Design review of the part built by this model. Coordinates are the model's own, in mm. Coordinates: 2 decimals unless noted, no trailing zeros. Loops run counter-clockwise (first coordinate to the right, second up) from the corner with the lowest first, then second, coordinate; pieces in that order, holes last. Notation, with made-up numbers: (-15.75, -30.75) -> (9.25, -30.75) arc R27 cw to (9.25, 2.25) -> close; hole circle Ø6 at (8, 16). An arc over 180 degrees is marked (long way). Answer as a JSON object with one key per item and string values.
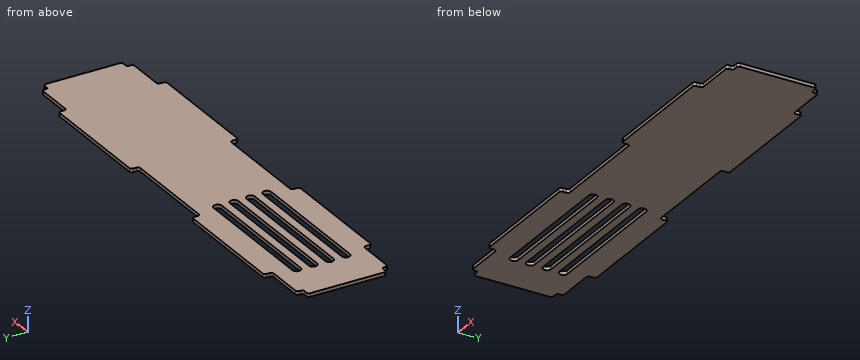
```python
from build123d import *

# Parameters (mm, degrees)
PAD_DEPTH = 1.8542


with BuildPart() as part:
    # Sketch (on Face54 of Binder001) → Pad (new body)
    with BuildSketch(Plane.XY.offset(-14.1418)):
        with BuildLine():
            Line((326.2352, 174.592), (328.0894, 174.592))
            ThreePointArc((329.2894, 173.392), (328.937928, 174.240528), (328.0894, 174.592))
            Line((329.2894, 173.392), (329.2894, 134.7706))
            ThreePointArc((328.0894, 133.5706), (328.937928, 133.922072), (329.2894, 134.7706))
            Line((328.0894, 133.5706), (326.2352, 133.5706))
            ThreePointArc((326.2352, 133.5706), (325.386672, 133.219128), (325.0352, 132.3706))
            Line((325.0352, 131.4813), (325.0352, 132.3706))
            ThreePointArc((323.8352, 130.2813), (324.683728, 130.632772), (325.0352, 131.4813))
            Line((304.7198, 130.2813), (323.8352, 130.2813))
            ThreePointArc((304.7198, 130.2813), (303.871272, 129.929828), (303.5198, 129.0813))
            Line((303.5198, 129.0813), (303.5198, 127.2271))
            ThreePointArc((302.3198, 126.0271), (303.168328, 126.378572), (303.5198, 127.2271))
            Line((241.3778, 126.0271), (302.3198, 126.0271))
            ThreePointArc((240.1778, 127.2271), (240.529272, 126.378572), (241.3778, 126.0271))
            Line((240.1778, 129.0813), (240.1778, 127.2271))
            ThreePointArc((240.1778, 129.0813), (239.826328, 129.929828), (238.9778, 130.2813))
            Line((187.7682, 130.2813), (238.9778, 130.2813))
            ThreePointArc((187.7682, 130.2813), (186.919672, 129.929828), (186.5682, 129.0813))
            Line((186.5682, 129.0813), (186.5682, 127.2271))
            ThreePointArc((185.3682, 126.0271), (186.216728, 126.378572), (186.5682, 127.2271))
            Line((124.6802, 126.0271), (185.3682, 126.0271))
            ThreePointArc((123.4802, 127.2271), (123.831672, 126.378572), (124.6802, 126.0271))
            Line((123.4802, 129.0813), (123.4802, 127.2271))
            ThreePointArc((123.4802, 129.0813), (123.128728, 129.929828), (122.2802, 130.2813))
            Line((122.2802, 130.2813), (103.1648, 130.2813))
            ThreePointArc((101.9648, 131.4813), (102.316272, 130.632772), (103.1648, 130.2813))
            Line((101.9648, 131.4813), (101.9648, 132.3706))
            ThreePointArc((101.9648, 132.3706), (101.613328, 133.219128), (100.7648, 133.5706))
            Line((100.7648, 133.5706), (98.9106, 133.5706))
            ThreePointArc((97.7106, 134.7706), (98.062072, 133.922072), (98.9106, 133.5706))
            Line((97.7106, 134.7706), (97.7106, 173.392))
            ThreePointArc((98.9106, 174.592), (98.062072, 174.240528), (97.7106, 173.392))
            Line((98.9106, 174.592), (100.7648, 174.592))
            ThreePointArc((100.7648, 174.592), (101.613328, 174.943472), (101.9648, 175.792))
            Line((101.9648, 175.792), (101.9648, 176.6813))
            ThreePointArc((103.1648, 177.8813), (102.316272, 177.529828), (101.9648, 176.6813))
            Line((103.1648, 177.8813), (122.2802, 177.8813))
            ThreePointArc((122.2802, 177.8813), (123.128728, 178.232772), (123.4802, 179.0813))
            Line((123.4802, 179.0813), (123.4802, 180.9355))
            ThreePointArc((124.6802, 182.1355), (123.831672, 181.784028), (123.4802, 180.9355))
            Line((124.6802, 182.1355), (185.3682, 182.1355))
            ThreePointArc((186.5682, 180.9355), (186.216728, 181.784028), (185.3682, 182.1355))
            Line((186.5682, 180.9355), (186.5682, 179.0813))
            ThreePointArc((186.5682, 179.0813), (186.919672, 178.232772), (187.7682, 177.8813))
            Line((238.9778, 177.8813), (187.7682, 177.8813))
            ThreePointArc((238.9778, 177.8813), (239.826328, 178.232772), (240.1778, 179.0813))
            Line((240.1778, 179.0813), (240.1778, 180.9355))
            ThreePointArc((241.3778, 182.1355), (240.529272, 181.784028), (240.1778, 180.9355))
            Line((241.3778, 182.1355), (302.3198, 182.1355))
            ThreePointArc((303.5198, 180.9355), (303.168328, 181.784028), (302.3198, 182.1355))
            Line((303.5198, 180.9355), (303.5198, 179.0813))
            ThreePointArc((303.5198, 179.0813), (303.871272, 178.232772), (304.7198, 177.8813))
            Line((304.7198, 177.8813), (323.8352, 177.8813))
            ThreePointArc((325.0352, 176.6813), (324.683728, 177.529828), (323.8352, 177.8813))
            Line((325.0352, 176.6813), (325.0352, 175.792))
            ThreePointArc((325.0352, 175.792), (325.386672, 174.943472), (326.2352, 174.592))
        make_face()
        with BuildLine():
            ThreePointArc((120.6, 143.367014), (118.457143, 141.224157), (120.6, 139.0813))
            Line((120.6, 139.0813), (189.4484, 139.0813))
            ThreePointArc((189.4484, 139.0813), (191.591257, 141.224157), (189.4484, 143.367014))
            Line((120.6, 143.367014), (189.4484, 143.367014))
        make_face(mode=Mode.SUBTRACT)
        with BuildLine():
            ThreePointArc((120.6, 151.938443), (118.457143, 149.795586), (120.6, 147.652729))
            Line((120.6, 147.652729), (189.4484, 147.652729))
            ThreePointArc((189.4484, 147.652729), (191.591257, 149.795586), (189.4484, 151.938443))
            Line((120.6, 151.938443), (189.4484, 151.938443))
        make_face(mode=Mode.SUBTRACT)
        with BuildLine():
            ThreePointArc((120.6, 160.509871), (118.457143, 158.367014), (120.6, 156.224157))
            Line((120.6, 156.224157), (189.4484, 156.224157))
            ThreePointArc((189.4484, 156.224157), (191.591257, 158.367014), (189.4484, 160.509871))
            Line((120.6, 160.509871), (189.4484, 160.509871))
        make_face(mode=Mode.SUBTRACT)
        with BuildLine():
            ThreePointArc((120.6, 169.0813), (118.457143, 166.938443), (120.6, 164.795586))
            Line((120.6, 164.795586), (189.4484, 164.795586))
            ThreePointArc((189.4484, 164.795586), (191.591257, 166.938443), (189.4484, 169.0813))
            Line((120.6, 169.0813), (189.4484, 169.0813))
        make_face(mode=Mode.SUBTRACT)
    extrude(amount=PAD_DEPTH)


solid = part.part
```
1) Clearance check with flat-ended pins moving along their axes: pin 1 Ø0.6 at (x, z) = (99.5, -13) entering from -Y; pin 2 Ø0.9 at (y, z) = (180, -13) entering from -X; pin 3 Ø1 at (y, z) = (176.5, -13.5) entering from +X. State where each tip first meets the part, or that it passes through.
Completed:
{"pin 1": "y = 133.57", "pin 2": "x = 123.48", "pin 3": "x = 325.04"}
2) Add section C-C, the plane x = 230. Give the boundary of the cut face in (y, z), and give its area (3 significant figures).
Completed:
{"outline": "(130.28, -14.14) -> (177.88, -14.14) -> (177.88, -12.29) -> (130.28, -12.29) -> close", "area": "88.3 mm²"}
3) Wall thickness on probe 1 along Y at (x, z) = (178, -13.5); probe 2 along X at (y, z) = (129, -13.5); probe 3 along Y at (x, z) = (230, -13.95): over which ranges is each line inside the solid? List them lowest first.
Completed:
{"probe 1": "126.03 to 139.08, 143.37 to 147.65, 151.94 to 156.22, 160.51 to 164.8, 169.08 to 182.14", "probe 2": "123.48 to 186.57, 240.18 to 303.52", "probe 3": "130.28 to 177.88"}
4) Add section B-B, the plane z = -13.4. Count the separate pieces of the cut face and the enclosed holes in it, and give its area (3 significant figures).
Completed:
{"separate pieces": "1", "enclosed holes": "4", "area": "10,800 mm²"}
5) Add section A-A, the plane x = 150.5. Give the boundary of the cut face in (y, z).
Completed:
{"outline": "(126.03, -14.14) -> (139.08, -14.14) -> (139.08, -12.29) -> (126.03, -12.29) -> close; (143.37, -14.14) -> (147.65, -14.14) -> (147.65, -12.29) -> (143.37, -12.29) -> close; (151.94, -14.14) -> (156.22, -14.14) -> (156.22, -12.29) -> (151.94, -12.29) -> close; (160.51, -14.14) -> (164.8, -14.14) -> (164.8, -12.29) -> (160.51, -12.29) -> close; (169.08, -14.14) -> (182.14, -14.14) -> (182.14, -12.29) -> (169.08, -12.29) -> close"}
